from build123d import *

# Parameters (mm, degrees)
BOSS_EXTRUDE1_DEPTH     = 10
BOSS_EXTRUDE1_2_DEPTH   = 10
SKETCH1_4_R             = 1.5
BOSS_EXTRUDE2_DEPTH     = 10.2
SKETCH2_R               = 10.5
CUT_EXTRUDE1_DEPTH      = 35.905730189
SKETCH2_3_R             = 12
CUT_EXTRUDE2_DEPTH      = 3
CUT_EXTRUDE3_DEPTH      = 1.5
LPATTERN2_COUNT         = 6
LPATTERN2_PITCH         = 3
MIRROR1_COPY_1_DEPTH    = 1.5
MIRROR1_COPY_2_DEPTH    = 1.5
MIRROR1_COPY_3_DEPTH    = 1.5
MIRROR1_COPY_4_DEPTH    = 1.5
MIRROR1_COPY_5_DEPTH    = 1.5
CUT_EXTRUDE4_REACH      = 44.359
CUT_EXTRUDE4_END_RADIUS = 10.5
SKETCH4_R               = 4
SKETCH5_R               = 1.5
CUT_EXTRUDE5_DEPTH      = 4


with BuildPart() as part:
    # Sketch1 → Boss-Extrude1 (new, symmetric)
    with BuildSketch(Plane(origin=(0, 0, 0), x_dir=(1, 0, 0), z_dir=(0, 1, 0))):
        with BuildLine():
            ThreePointArc((17.204650534, 14.5), (0, 22.5), (-17.204650534, 14.5))
            Line((-17.204650534, 14.5), (-17.204650534, 8.062257748))
            ThreePointArc((-17.204650534, 8.062257748), (0, 19), (17.204650534, 8.062257748))
            Line((17.204650534, 8.062257748), (17.204650534, 14.5))
        make_face()
    extrude(amount=BOSS_EXTRUDE1_DEPTH, both=True)



with BuildPart() as body_2:
    # Sketch1 → Boss-Extrude1 2 (new, symmetric)
    with BuildSketch(Plane(origin=(0, 0, 0), x_dir=(1, 0, 0), z_dir=(0, 1, 0))):
        with BuildLine():
            ThreePointArc((17.204650534, -8.062257748), (0, -19), (-17.204650534, -8.062257748))
            Line((-17.204650534, -8.062257748), (-17.204650534, -14.5))
            ThreePointArc((-17.204650534, -14.5), (0, -22.5), (17.204650534, -14.5))
            Line((17.204650534, -14.5), (17.204650534, -8.062257748))
        make_face()
    extrude(amount=BOSS_EXTRUDE1_2_DEPTH, both=True)


with BuildPart() as part_1:
    add(part.part)

    add(body_2.part)  # Boss-Extrude2 merges body 2
    # Sketch1<4> → Boss-Extrude2 (add, symmetric)
    with BuildSketch(Plane(origin=(0, 0, 0), x_dir=(1, 0, 0), z_dir=(0, 1, 0))):
        with BuildLine():
            ThreePointArc((17.204650534, 8.062257748), (0, 19), (-17.204650534, 8.062257748))
            Line((-17.204650534, 8.062257748), (-17.204650534, -8.062257748))
            ThreePointArc((-17.204650534, -8.062257748), (0, -19), (17.204650534, -8.062257748))
            Line((17.204650534, -8.062257748), (17.204650534, 8.062257748))
        make_face()
        with Locations(Location((-13.856406461, -8, 0), (0, 0, 270))):
            Circle(SKETCH1_4_R, mode=Mode.SUBTRACT)
        with Locations(Location((0, -16, 0), (0, 0, 270))):
            Circle(SKETCH1_4_R, mode=Mode.SUBTRACT)
        with Locations(Location((13.856406461, -8, 0), (0, 0, 270))):
            Circle(SKETCH1_4_R, mode=Mode.SUBTRACT)
        with Locations(Location((-13.856406461, 8, 0), (0, 0, 270))):
            Circle(SKETCH1_4_R, mode=Mode.SUBTRACT)
        with Locations(Location((13.856406461, 8, 0), (0, 0, 270))):
            Circle(SKETCH1_4_R, mode=Mode.SUBTRACT)
        with Locations(Location((0, 16, 0), (0, 0, 270))):
            Circle(SKETCH1_4_R, mode=Mode.SUBTRACT)
    extrude(amount=BOSS_EXTRUDE2_DEPTH, both=True)

    # Sketch2 → Cut-Extrude1 (cut, through all)
    with BuildSketch(Plane(origin=(0, 10.2, 0), x_dir=(1, 0, 0), z_dir=(0, 1, 0))):
        with Locations(Location((0, 0, 0), (0, 0, 270))):
            Circle(SKETCH2_R)
    extrude(amount=-CUT_EXTRUDE1_DEPTH, mode=Mode.SUBTRACT)

    # Sketch2<3> → Cut-Extrude2 (cut)
    with BuildSketch(Plane(origin=(0, 10.2, 0), x_dir=(1, 0, 0), z_dir=(0, 1, 0))):
        with Locations(Location((0, 0, 0), (0, 0, 270))):
            Circle(SKETCH2_3_R)
    extrude(amount=-CUT_EXTRUDE2_DEPTH, mode=Mode.SUBTRACT)

    # Sketch3 → Cut-Extrude3 (cut)
    with BuildSketch(Plane(origin=(0, 8.5, 0), x_dir=(1, 0, 0), z_dir=(0, 1, 0))):
        with BuildLine():
            Line((17.204650534, 8.062257748), (17.204650534, 14.5))
            ThreePointArc((17.204650534, 14.5), (0, 22.5), (-17.204650534, 14.5))
            Line((-17.204650534, 14.5), (-17.204650534, 8.062257748))
            ThreePointArc((-17.204650534, 8.062257748), (0, 19), (17.204650534, 8.062257748))
        make_face()
    cut_extrude3 = extrude(amount=-CUT_EXTRUDE3_DEPTH, mode=Mode.SUBTRACT)

    # LPattern2: Cut-Extrude3 ×6
    with Locations(*[(0, -i * LPATTERN2_PITCH, 0) for i in range(1, LPATTERN2_COUNT)]):
        add(cut_extrude3, mode=Mode.SUBTRACT)

    # Mirror1: Cut-Extrude3 across plane
    add(cut_extrude3.mirror(Plane.XY), mode=Mode.SUBTRACT)

    # Mirror1 copy 1 sketch → Mirror1 copy 1 (cut)
    with BuildSketch(Plane(origin=(0, 5.5, 0), x_dir=(1, 0, 0), z_dir=(0, 1, 0))):
        with BuildLine():
            Line((17.204650534, -8.062257748), (17.204650534, -14.5))
            ThreePointArc((17.204650534, -14.5), (0, -22.5), (-17.204650534, -14.5))
            Line((-17.204650534, -14.5), (-17.204650534, -8.062257748))
            ThreePointArc((-17.204650534, -8.062257748), (0, -19), (17.204650534, -8.062257748))
        make_face()
    extrude(amount=-MIRROR1_COPY_1_DEPTH, mode=Mode.SUBTRACT)

    # Mirror1 copy 2 sketch → Mirror1 copy 2 (cut)
    with BuildSketch(Plane(origin=(0, 2.5, 0), x_dir=(1, 0, 0), z_dir=(0, 1, 0))):
        with BuildLine():
            Line((17.204650534, -8.062257748), (17.204650534, -14.5))
            ThreePointArc((17.204650534, -14.5), (0, -22.5), (-17.204650534, -14.5))
            Line((-17.204650534, -14.5), (-17.204650534, -8.062257748))
            ThreePointArc((-17.204650534, -8.062257748), (0, -19), (17.204650534, -8.062257748))
        make_face()
    extrude(amount=-MIRROR1_COPY_2_DEPTH, mode=Mode.SUBTRACT)

    # Mirror1 copy 3 sketch → Mirror1 copy 3 (cut)
    with BuildSketch(Plane(origin=(0, -0.5, 0), x_dir=(1, 0, 0), z_dir=(0, 1, 0))):
        with BuildLine():
            Line((17.204650534, -8.062257748), (17.204650534, -14.5))
            ThreePointArc((17.204650534, -14.5), (0, -22.5), (-17.204650534, -14.5))
            Line((-17.204650534, -14.5), (-17.204650534, -8.062257748))
            ThreePointArc((-17.204650534, -8.062257748), (0, -19), (17.204650534, -8.062257748))
        make_face()
    extrude(amount=-MIRROR1_COPY_3_DEPTH, mode=Mode.SUBTRACT)

    # Mirror1 copy 4 sketch → Mirror1 copy 4 (cut)
    with BuildSketch(Plane(origin=(0, -3.5, 0), x_dir=(1, 0, 0), z_dir=(0, 1, 0))):
        with BuildLine():
            Line((17.204650534, -8.062257748), (17.204650534, -14.5))
            ThreePointArc((17.204650534, -14.5), (0, -22.5), (-17.204650534, -14.5))
            Line((-17.204650534, -14.5), (-17.204650534, -8.062257748))
            ThreePointArc((-17.204650534, -8.062257748), (0, -19), (17.204650534, -8.062257748))
        make_face()
    extrude(amount=-MIRROR1_COPY_4_DEPTH, mode=Mode.SUBTRACT)

    # Mirror1 copy 5 sketch → Mirror1 copy 5 (cut)
    with BuildSketch(Plane(origin=(0, -6.5, 0), x_dir=(1, 0, 0), z_dir=(0, 1, 0))):
        with BuildLine():
            Line((17.204650534, -8.062257748), (17.204650534, -14.5))
            ThreePointArc((17.204650534, -14.5), (0, -22.5), (-17.204650534, -14.5))
            Line((-17.204650534, -14.5), (-17.204650534, -8.062257748))
            ThreePointArc((-17.204650534, -8.062257748), (0, -19), (17.204650534, -8.062257748))
        make_face()
    extrude(amount=-MIRROR1_COPY_5_DEPTH, mode=Mode.SUBTRACT)

    # Cut-Extrude4: up to this cylinder (the profile starts outside it)
    cut_extrude4_end = Plane(origin=(0, 0, 0), z_dir=(0, 1, 0)) * Cylinder(CUT_EXTRUDE4_END_RADIUS, 110.718, mode=Mode.PRIVATE)
    # Sketch4 → Cut-Extrude4 (cut, up to the surface)
    with BuildSketch(Plane(origin=(17.204650534, 0, 0), x_dir=(0, 0, -1), z_dir=(1, 0, 0)), mode=Mode.PRIVATE) as cut_extrude4_sk1:
        Circle(SKETCH4_R)
    cut_extrude4_tool1 = extrude(cut_extrude4_sk1.sketch, amount=-CUT_EXTRUDE4_REACH, mode=Mode.PRIVATE) - cut_extrude4_end
    add(cut_extrude4_tool1.solids().sort_by_distance((17.204651, 0, 0))[0], mode=Mode.SUBTRACT)

    # Sketch5 → Cut-Extrude5 (cut)
    with BuildSketch(Plane(origin=(17.204650534, 0, 0), x_dir=(0, 0, -1), z_dir=(1, 0, 0))):
        with Locations((4.949747468, 4.949747468)):
            Circle(SKETCH5_R)
        with Locations((4.949747468, -4.949747468)):
            Circle(SKETCH5_R)
        with Locations((-4.949747468, -4.949747468)):
            Circle(SKETCH5_R)
        with Locations((-4.949747468, 4.949747468)):
            Circle(SKETCH5_R)
    cut_extrude5 = extrude(amount=-CUT_EXTRUDE5_DEPTH, mode=Mode.SUBTRACT)

    # Sketch6 → Cut-Revolve1 (revolve, cut)
    with BuildSketch(Plane(origin=(0, 0.2, 0), x_dir=(1, 0, 0), z_dir=(0, 1, 0)), mode=Mode.PRIVATE) as cut_revolve1_sk:
        Polygon((-17.204650534, -3), (-14.704650534, -3), (-11.704650534, 0), (-17.204650534, 0), align=None)
    revolve(cut_revolve1_sk.sketch.rotate(Axis((-11.704650534, 0.2, 0), (-1, 0, 0)), 180), axis=Axis((-11.704650534, 0.2, 0), (-1, 0, 0)), mode=Mode.SUBTRACT)

    # Mirror2: Cut-Extrude5 across plane
    add(cut_extrude5.mirror(Plane(origin=(0, 0, 0), x_dir=(0, 0, 1), z_dir=(1, 0, 0))), mode=Mode.SUBTRACT)


solid = part_1.part
Could you check a few things on this model? Use its own coordinates, in mm. A direction names the side the tool comes from. Coordinates: 2 decimals unless noted, no trailing zeros. Loops run counter-clockwise (first coordinate to the right, second up) from the corner with the lowest first, then second, coordinate; pieces in that order, holes last.
1. For faces 1 (the face through (0, 2.5, -20)), 2 (the face through (0, 10, -20)), 3 (the face through (0, 5.5, 20)), which set-ups out of +Z, -Z, +X, -X, +Y, -Y let a thin tool reach every point of the face, with its end or its side?
2. Imagine slicing it at A-A (x = 0). Give the number of separate pieces and of enclosed holes in the cut face, and give its area (3 significant figures).
3. Imagine slicing it at B-B (z = 4.5). Please give me the cut outline in (x, y), and give its area (3 significant figures).
4. I need wall thicknesses on L1, parallel to X at y = 8.25, z = 0; L2, parallel to Z at x = -1, y = 6.75; L3, parallel to Z at x = 13, y = 0. Which ranges of each line are inside material? Lowest first, please.
5. For P1, Ø5, axis at y = 0, z = 0, coming from the -X side; P2, Ø1.5, axis at x = 2, y = 1, coming from the +Z side; P3, Ø1, axis at x = 12.5, y = -8, coming from the +Z side, each with a flat end and sliding along its axis, tell me the tip position at first contact or that it passes through.
6. We'd pull the mould along Z, two halves only. Please class faces 4 (the face through (0.07, -0.14, -17.5)), 5 (the face through (-0.3, -2.7, 22.5)), 6 (the face through (0, 2, -19)), 7 (the face through (0, -3.5, -20)): released by +Z, released by -Z, zero draft, split by the parting line, or undercut.
Computed values:
1. face 1: -Z
1. face 2: -Z, +Y
1. face 3: +Z
2. separate pieces: 4
2. enclosed holes: 0
2. area: 292 mm2
3. outline: (-17.2, -10.2) - (-9.49, -10.2) - (-9.49, 7.2) - (-11.12, 7.2) - (-11.12, 10.2) - (-17.2, 10.2) - (-17.2, 6.38) - (-13.2, 6.38) - (-13.2, 3.52) - (-17.2, 3.52) - (-17.2, -3.52) - (-13.2, -3.52) - (-13.2, -6.38) - (-17.2, -6.38) - close; (9.49, -10.2) - (17.2, -10.2) - (17.2, -6.38) - (13.2, -6.38) - (13.2, -3.52) - (17.2, -3.52) - (17.2, 3.52) - (13.2, 3.52) - (13.2, 6.38) - (17.2, 6.38) - (17.2, 10.2) - (11.12, 10.2) - (11.12, 7.2) - (9.49, 7.2) - close
3. area: 259 mm2
4. L1: x = -17.2 to -12, 12 to 17.2
4. L2: z = -22.48 to -17.12, -14.88 to -10.45, 10.45 to 14.88, 17.12 to 22.48
4. L3: z = -18.36 to -9.23, -6.77 to -4, 4 to 6.77, 9.23 to 18.36
5. P1: stops at x = -14.4
5. P2: stops at z = 22.47
5. P3: stops at z = 19.03
6. face 4: undercut
6. face 5: released by +Z
6. face 6: released by -Z
6. face 7: zero draft
